Geometry: final body of the model. Coordinates: model frame, mm. Face numbers are marked on the shaded views. A direction names the side the tool comes from. Give positions to 0.01 mm unless a question says otherwise; leave off trailing zeros. Write each loop counter-clockwise with the first axis right and the second up, starting at its lowest first coordinate (ties: lowest second). Pieces come first, ordered by that corner, then holes. Notation, with made-up numbers: M 48,88.25 L 93,88.25 A25 cw 93,103.25 Z; hole C -19.5,-14 d3. An arc over 180 degrees is marked long. Use a Markdown table: item, result. Add a question column.
1) Draft query along Z for the marked faces 4, 5, 6 and 7. Return one class per face: +Z half, -Z half, draft (parallel to the pull), parting line (faces both ways), or undercut.
2) Pin query (flat end, axial travel): pin 1 (1.5 mm diameter, centred on x = 34.5, z = -24, fed in from +Y); pin 2 (5 mm diameter, centred on y = 10, z = -27.5, fed in from +X); pin 3 (2.5 mm diameter, centred on x = 57.5, y = 9.5, fed in from -Z). Return the tip coordinate at first contact, or that it passes through.
3) Section B-B on x = 57. Return the cut outline in (y, z).
4) Line query: line 1 (Z direction, x = 28.5, y = 6); line 2 (X direction, y = 14.5, z = -27.5); line 3 (Y direction, x = 57, z = -0.6). Output: solid intervals per line, ascending.
5) Section C-C on x = 40. Return the cut outline in (y, z).
6) Set-up query: the marked faces 1, 2 and 3. Return all of +Z, -Z, +X, -X, +Y, -Y with unobstructed straight access to the full face (end or side cutting, diameter ignored); none if empty.
7) Section A-A on y = 9.5. Return the cut outline in (x, z), then the cut area to 3 significant figures.
8) Section D-D on z = -23. Return the cut outline in (x, y).
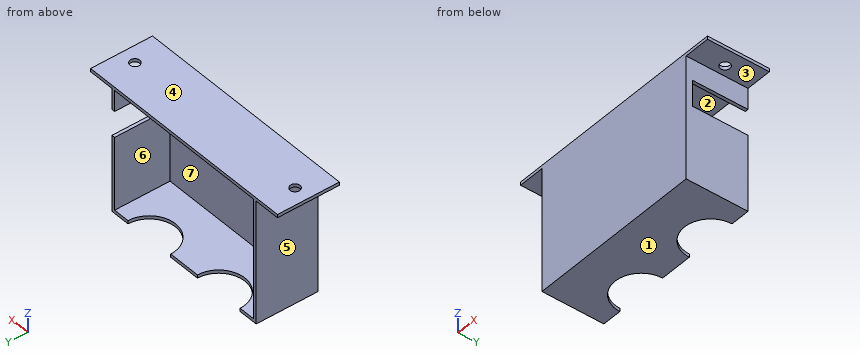
```python
from build123d import *

# Parameters (mm, degrees)
SKETCH1_W           = 52
SKETCH1_H           = 37
BOSS_EXTRUDE1_DEPTH = 19
CUT_EXTRUDE1_REACH  = 41
SKETCH2_R           = 1.5
SKETCH3_W           = 52
SKETCH3_H           = 37
BOSS_EXTRUDE2_DEPTH = 2
CUT_EXTRUDE2_REACH  = 41
SKETCH4_R           = 8
SKETCH5_W           = 8
SKETCH5_H           = 17
CUT_EXTRUDE3_DEPTH  = 1


with BuildPart() as part:
    # Sketch1 → Boss-Extrude1 (new body)
    with BuildSketch(Plane(origin=(0, 0, 0), x_dir=(1, 0, 0), z_dir=(0, 1, 0))):
        Polygon((54, 0), (62, 0), (62, 1), (54, 1), (54, 39), (0, 39), (0, 1), (-8, 1), (-8, 0), (0, 0), align=None)
        with Locations((27, 19.5)):
            Rectangle(SKETCH1_W, SKETCH1_H, mode=Mode.SUBTRACT)
    extrude(amount=BOSS_EXTRUDE1_DEPTH)

    # Sketch2 → Cut-Extrude1 (cut, up to next)
    with BuildSketch(Plane.XY, mode=Mode.PRIVATE) as cut_extrude1_sk1:
        with Locations((-3, 9.5)):
            Circle(SKETCH2_R)
    cut_extrude1_tool1 = extrude(cut_extrude1_sk1.sketch, amount=-CUT_EXTRUDE1_REACH, mode=Mode.PRIVATE) & part.part
    add(cut_extrude1_tool1.solids().sort_by_distance((-3, 9.5, 0))[0], mode=Mode.SUBTRACT)
    # Sketch2 → Cut-Extrude1 (cut, up to next)
    with BuildSketch(Plane.XY, mode=Mode.PRIVATE) as cut_extrude1_sk2:
        with Locations((57, 9.5)):
            Circle(SKETCH2_R)
    cut_extrude1_tool2 = extrude(cut_extrude1_sk2.sketch, amount=-CUT_EXTRUDE1_REACH, mode=Mode.PRIVATE) & part.part
    add(cut_extrude1_tool2.solids().sort_by_distance((57, 9.5, 0))[0], mode=Mode.SUBTRACT)

    # Sketch3 → Boss-Extrude2 (add)
    with BuildSketch(Plane(origin=(0, 0, 0), x_dir=(1, 0, 0), z_dir=(0, 1, 0))):
        with Locations((27, 19.5)):
            Rectangle(SKETCH3_W, SKETCH3_H)
    extrude(amount=BOSS_EXTRUDE2_DEPTH)

    # Sketch4 → Cut-Extrude2 (cut, up to next)
    with BuildSketch(Plane(origin=(0, 0, -39), x_dir=(-1, 0, 0), z_dir=(0, 0, -1)), mode=Mode.PRIVATE) as cut_extrude2_sk1:
        with Locations((-14, 19)):
            Circle(SKETCH4_R)
    cut_extrude2_tool1 = extrude(cut_extrude2_sk1.sketch, amount=-CUT_EXTRUDE2_REACH, mode=Mode.PRIVATE) & part.part
    add(cut_extrude2_tool1.solids().sort_by_distance((14, 19, -39))[0], mode=Mode.SUBTRACT)
    # Sketch4 → Cut-Extrude2 (cut, up to next)
    with BuildSketch(Plane(origin=(0, 0, -39), x_dir=(-1, 0, 0), z_dir=(0, 0, -1)), mode=Mode.PRIVATE) as cut_extrude2_sk2:
        with Locations((-40, 19)):
            Circle(SKETCH4_R)
    cut_extrude2_tool2 = extrude(cut_extrude2_sk2.sketch, amount=-CUT_EXTRUDE2_REACH, mode=Mode.PRIVATE) & part.part
    add(cut_extrude2_tool2.solids().sort_by_distance((40, 19, -39))[0], mode=Mode.SUBTRACT)

    # Sketch5 → Cut-Extrude3 (cut)
    with BuildSketch(Plane(origin=(54, 0, 0), x_dir=(0, 0, -1), z_dir=(1, 0, 0))):
        with Locations((11.5, 10.5)):
            Rectangle(SKETCH5_W, SKETCH5_H)
    extrude(amount=-CUT_EXTRUDE3_DEPTH, mode=Mode.SUBTRACT)


solid = part.part
```
Found:
| question | item | result |
|---|---|---|
| 1 | face 4 | +Z half |
| 1 | face 5 | draft |
| 1 | face 6 | undercut |
| 1 | face 7 | undercut |
| 2 | pin 1 | y = 2 |
| 2 | pin 2 | x = 54 |
| 2 | pin 3 | z = -1 |
| 3 | outline | M 0,-1 L 8,-1 L 8,0 L 0,0 Z; M 11,-1 L 19,-1 L 19,0 L 11,0 Z |
| 4 | line 1 | -39 to -38, -1 to 0 |
| 4 | line 2 | 0 to 1, 53 to 54 |
| 4 | line 3 | 0 to 8, 11 to 19 |
| 5 | outline | M 0,-39 L 11,-39 L 11,-38 L 2,-38 L 2,-1 L 19,-1 L 19,0 L 0,0 Z |
| 6 | face 1 | -Z, +X, -X, +Y, -Y |
| 6 | face 2 | +Y |
| 6 | face 3 | -Z, +X, +Y, -Y |
| 7 | outline | M -8,-1 L -4.5,-1 L -4.5,0 L -8,0 Z; M -1.5,-1 L 0,-1 L 0,-39 L 54,-39 L 54,-15.5 L 53,-15.5 L 53,-38 L 1,-38 L 1,-1 L 53,-1 L 53,-7.5 L 54,-7.5 L 54,-1 L 55.5,-1 L 55.5,0 L -1.5,0 Z; M 58.5,-1 L 62,-1 L 62,0 L 58.5,0 Z |
| 7 | area | 184 mm² |
| 8 | outline | M 0,0 L 54,0 L 54,19 L 53,19 L 53,2 L 1,2 L 1,19 L 0,19 Z |
